Could you check a few things on this model? Use its own coordinates, in mm. A direction names the side the tool comes from. Coordinates: 2 decimals unless noted, no trailing zeros. Order: outer loops, then holes, each group sorted by start corner. A loop starts at its lowest first (then second) coordinate and runs counter-clockwise, first axis right, second up. Notation, with made-up numbers: M 74.5,53 L 119.5,53 A25 ccw 119.5,75 Z; hole C 85.5,30.5 d5. An arc over 180 degrees is marked long. Put each result on its own line as item: value. Start each with the question number.
Autodesk Inventor part; units mm, degrees
ref_plane "YZ Plane" through (0, 0, 0) normal (1, 0, 0) x (0, 1, 0)
ref_plane "XZ Plane" through (0, 0, 0) normal (0, 1, 0) x (-1, 0, 0)
ref_plane "XY Plane" through (0, 0, 0) normal (0, 0, 1) x (1, 0, 0)
sketch "Sketch1" plane through (0, 0, 0) normal (0, 0, 1) x (1, 0, 0)
  line L0 (-33.5, -13) -> (33.5, -13) construction
  line L1 (33.5, -13) -> (33.5, 13) construction
  line L2 (33.5, 13) -> (-33.5, 13) construction
  line L3 (-33.5, 13) -> (-33.5, -13) construction
  line L4 (-33.5, -13) -> (33.5, 13) construction
  line L5 (33.5, -13) -> (-33.5, 13) construction
  arc A0 (-33.5, 19) -> (-39.3825, 11.8182) centre (-33.5, 13) ccw
  arc A1 (-39.3825, -11.8182) -> (-33.5, -19) centre (-33.5, -13) ccw
  arc A2 (33.5, -19) -> (39.3825, -11.8182) centre (33.5, -13) ccw
  arc A3 (39.3825, 11.8182) -> (33.5, 19) centre (33.5, 13) ccw
  arc A4 (-39.3825, -11.8182) -> (-39.3825, 11.8182) centre (-98.207, 0) ccw
  arc A5 (39.3825, 11.8182) -> (39.3825, -11.8182) centre (98.207, 0) ccw
  line L6 (-33.5, 19) -> (33.5, 19)
  line L7 (-33.5, -19) -> (33.5, -19)
  point P0 (0, 0)
  dimension "d0" = 67
  dimension "d1" = 26
  dimension "d2" = 6
  dimension "d3" = 60
extrude "Extrusion1" add sketch "Sketch1" along normal blind 6
sketch "Sketch2" plane through (0, 0, 0) normal (1, 0, 0) x (0, 1, 0)
  line L0 (19, 6) -> (11.8182, 6) construction
  line L1 (19, 6) -> (7, 49)
  line L2 (7, 49) -> (1, 49)
  line L3 (1, 49) -> (-19, 6)
  line L4 (19, 6) -> (11.8182, 6) construction
  line L5 (11.8182, 6) -> (-11.8182, 6) construction
  line L6 (-11.8182, 6) -> (-19, 6) construction
  line L7 (-19, 6) -> (-11.8182, 6) construction
  line L8 (-11.8182, 6) -> (11.8182, 6) construction
  line L9 (11.8182, 6) -> (19, 6) construction
  line L10 (19, 6) -> (-19, 6)
  point P0 (0, 0)
  dimension "d7" = 12
  dimension "d8" = 43
  dimension "d9" = 6
extrude "Extrusion2" add sketch "Sketch2" along normal mid plane 55
sketch "Sketch3" plane through (-27.5, 1, 49) normal (0, 0, 1) x (1, 0, 0)
  line L0 (0, 0) -> (55, 0)
  line L1 (55, 6) -> (55, 0)
  line L2 (0, 6) -> (55, 6)
  line L3 (0, 0) -> (0, 6)
  line L4 (0, 6) -> (55, 6)
  line L5 (61, 18) -> (-6, 18)
  line L6 (4, 6) -> (51, 6)
  line L7 (51, 6) -> (51, 18)
  line L8 (51, 18) -> (4, 18)
  line L9 (4, 18) -> (4, 6)
  line L10 (0, 0) -> (55, 0)
  line L11 (-6, -20) -> (61, -20)
  line L12 (4, 0) -> (51, 0)
  line L13 (51, 0) -> (51, -20)
  line L14 (51, -20) -> (4, -20)
  line L15 (4, -20) -> (4, 0)
  point P0 (27.5, -1)
  dimension "d12" = 4
  dimension "d13" = 4
extrude "Extrusion3" cut sketch "Sketch3" against normal up to surface (43 mm away) contours L0 L13 L11 L15 | L9 L5 L7 L2
sketch "Sketch4" plane through (-23.5, 7, 49) normal (0, 1, 0) x (1, 0, 0)
  arc A0 (36.54, 17.5059) -> (10.46, 17.5059) centre (23.5, 21) ccw
  line L0 (47, 43) -> (0, 43)
  line L1 (57, 49) -> (-10, 49)
  line L2 (36.54, 17.5059) -> (31.8493, 0)
  line L3 (31.8493, 0) -> (15.1507, 0)
  line L4 (15.1507, 0) -> (10.46, 17.5059)
  line L5 (0, 0) -> (47, 0)
  arc A1 (10.46, 17.5059) -> (36.54, 17.5059) centre (23.5, 21) ccw construction
  point P0 (23.5, 49)
  point P1 (23.5, 49)
  point P2 (23.5, 0)
  point P3 (23.5, 49)
  dimension "d16" = 27
  dimension "d17" = 22
  dimension "d18" = 30
extrude "Extrusion4" cut sketch "Sketch4" against normal blind 55
fillet "Fillet1" radius 5 2 edges at (8.3493, 4, 49) (-8.3493, 4, 49)
sketch "Sketch5" plane through (-23.5, 7, 6) normal (0, 1, 0) x (1, 0, 0)
  arc A0 (36.54, -25.4941) -> (10.46, -25.4941) centre (23.5, -22) ccw
  line L0 (8, -6.5) -> (39, -6.5)
  line L1 (39, -6.5) -> (39, -37.5)
  line L2 (39, -37.5) -> (8, -37.5)
  line L3 (8, -37.5) -> (8, -6.5)
  line L4 (8, -6.5) -> (39, -37.5) construction
  line L5 (39, -6.5) -> (8, -37.5) construction
  point P0 (23.5, 6)
  dimension "d22" = 31
  dimension "d23" = 31
hole "Hole1" at (-15.5, 7, 12.5) at (15.5, 7, 12.5) at (15.5, 7, 43.5) at (-15.5, 7, 43.5) direction (0, -1, 0) diameter 4 end through all
sketch "Sketch6" plane through (0, 0, 0) normal (0, 0, -1) x (-1, 0, 0)
  arc A0 (-33.5, -19) -> (-32.6299, -18.9366) centre (-33.5, -13) ccw
  arc A1 (32.6299, -18.9366) -> (-32.6299, -18.9366) centre (0, -241.558) ccw
  arc A2 (32.6299, -18.9366) -> (33.5, -19) centre (33.5, -13) ccw
  line L0 (-33.5, -19) -> (33.5, -19)
  arc A3 (33.5, -19) -> (39.3825, -11.8182) centre (33.5, -13) ccw
  arc A4 (-39.3825, -11.8182) -> (-33.5, -19) centre (-33.5, -13) ccw
  point P0 (0, 0)
  dimension "d31" = 225
extrude "Extrusion5" cut sketch "Sketch6" against normal blind 55
sketch "Sketch7" plane through (0, 0, 0) normal (0, 0, -1) x (-1, 0, 0)
  line L0 (-33.5, -13) -> (33.5, -13) construction
  line L1 (33.5, -13) -> (33.5, 13) construction
  line L2 (33.5, 13) -> (-33.5, 13) construction
  line L3 (-33.5, 13) -> (-33.5, -13) construction
  line L4 (-33.5, -13) -> (33.5, 13) construction
  line L5 (33.5, -13) -> (-33.5, 13) construction
  arc A0 (-39.3825, -11.8182) -> (-32.6299, -18.9366) centre (-33.5, -13) ccw construction
  arc A1 (32.6299, -18.9366) -> (-32.6299, -18.9366) centre (0, -241.558) ccw construction
  arc A2 (32.6299, -18.9366) -> (39.3825, -11.8182) centre (33.5, -13) ccw construction
  arc A3 (39.3825, 11.8182) -> (39.3825, -11.8182) centre (98.207, 0) ccw construction
  arc A4 (39.3825, 11.8182) -> (33.5, 19) centre (33.5, 13) ccw construction
  line L6 (-33.5, 19) -> (33.5, 19) construction
  arc A5 (-33.5, 19) -> (-39.3825, 11.8182) centre (-33.5, 13) ccw construction
  arc A6 (-39.3825, -11.8182) -> (-39.3825, 11.8182) centre (-98.207, 0) ccw construction
  point P0 (0, 0)
  point P1 (0, 0)
  dimension "d34" = 67
  dimension "d35" = 26
hole "Hole2" at (33.5, 13, 0) at (33.5, -13, 0) at (-33.5, -13, 0) at (-33.5, 13, 0) direction (0, 0, 1) diameter 4 depth 14.2 tip angle 118
sketch "Sketch8" plane through (0, 0, 6) normal (0, 0, 1) x (1, 0, 0)
  circle A0 centre (-33.5, -13) radius 2
  circle A1 centre (-33.5, 13) radius 2
  arc A2 (-39.3825, -11.8182) -> (-32.6299, -18.9366) centre (-33.5, -13) ccw
  arc A3 (-27.5, -18.2449) -> (-32.6299, -18.9366) centre (0, -241.558) ccw
  line L0 (-27.5, -18.2449) -> (-27.5, 19)
  line L1 (-27.5, 19) -> (-33.5, 19)
  arc A4 (-33.5, 19) -> (-39.3825, 11.8182) centre (-33.5, 13) ccw
  arc A5 (-39.3825, -11.8182) -> (-39.3825, 11.8182) centre (-98.207, 0) ccw
  circle A6 centre (33.5, 13) radius 2
  circle A7 centre (33.5, -13) radius 2
  arc A8 (32.6299, -18.9366) -> (39.3825, -11.8182) centre (33.5, -13) ccw
  arc A9 (39.3825, 11.8182) -> (39.3825, -11.8182) centre (98.207, 0) ccw
  arc A10 (39.3825, 11.8182) -> (33.5, 19) centre (33.5, 13) ccw
  line L2 (33.5, 19) -> (27.5, 19)
  line L3 (27.5, 19) -> (27.5, -18.2449)
  arc A11 (32.6299, -18.9366) -> (27.5, -18.2449) centre (0, -241.558) ccw
  line L4 (-30.1519, 11.067) -> (-33.5, 9.134)
  line L5 (-33.5, 9.134) -> (-36.8481, 11.067)
  line L6 (-36.8481, 11.067) -> (-36.8481, 14.933)
  line L7 (-36.8481, 14.933) -> (-33.5, 16.866)
  line L8 (-33.5, 16.866) -> (-30.1519, 14.933)
  line L9 (-30.1519, 14.933) -> (-30.1519, 11.067)
  line L10 (-30.1519, -14.933) -> (-33.5, -16.866)
  line L11 (-33.5, -16.866) -> (-36.8481, -14.933)
  line L12 (-36.8481, -14.933) -> (-36.8481, -11.067)
  line L13 (-36.8481, -11.067) -> (-33.5, -9.134)
  line L14 (-33.5, -9.134) -> (-30.1519, -11.067)
  line L15 (-30.1519, -11.067) -> (-30.1519, -14.933)
  line L16 (36.8481, -14.933) -> (33.5, -16.866)
  line L17 (33.5, -16.866) -> (30.1519, -14.933)
  line L18 (30.1519, -14.933) -> (30.1519, -11.067)
  line L19 (30.1519, -11.067) -> (33.5, -9.134)
  line L20 (33.5, -9.134) -> (36.8481, -11.067)
  line L21 (36.8481, -11.067) -> (36.8481, -14.933)
  line L22 (36.8481, 11.067) -> (33.5, 9.134) construction
  line L23 (33.5, 9.134) -> (30.1519, 11.067) construction
  line L24 (30.1519, 11.067) -> (30.1519, 14.933) construction
  line L25 (30.1519, 14.933) -> (33.5, 16.866) construction
  line L26 (33.5, 16.866) -> (36.8481, 14.933) construction
  line L27 (36.8481, 14.933) -> (36.8481, 11.067) construction
  arc A12 (30.1519, 14.933) -> (33.5, 16.866) centre (30.075, 18.9323) ccw
  arc A13 (33.5, 16.866) -> (36.8481, 14.933) centre (36.925, 18.9323) ccw
  arc A14 (36.8481, 11.067) -> (33.5, 9.134) centre (36.925, 7.0677) ccw
  arc A15 (33.5, 9.134) -> (30.1519, 11.067) centre (30.075, 7.0677) ccw
  arc A16 (30.1519, 11.067) -> (30.1519, 14.933) centre (26.65, 13) ccw
  arc A17 (36.8481, 14.933) -> (36.8481, 11.067) centre (40.35, 13) ccw
  point P0 (0, 0)
  dimension "d44" = 6.6962
  dimension "d47" = 4
  dimension "d48" = 4
  dimension "d49" = 4
  dimension "d50" = 4
  dimension "d51" = 4
  dimension "d52" = 4
  dimension "d53" = 5.7
extrude "Extrusion6" cut sketch "Sketch8" against normal blind 3 contours A12 A13 A17 A14 A15 A16
pattern_linear "Rectangular Pattern1" count 2 spacing 67 along (-1, 0, 0) count 2 spacing 26 along (0, -1, 0) of "Extrusion6"
equation "\"d13\" = d12"
properties part number "Y Motor Mount" material "ABS Plastic"
Item 1: For pin 1 Ø7.5 at (x, y) = (34.5, 14) entering from +Z; pin 2 Ø13 at (y, z) = (12, 34) entering from +X; pin 3 Ø9.5 at (y, z) = (14.5, 36.5) entering from -X, each with a flat end and sliding along its axis, tell me the tip position at first contact or that it passes through.
Item 2: I need wall thicknesses on probe 1 along X at (y, z) = (13, 1.05); probe 2 along Y at (x, z) = (33.5, 1.25); probe 3 along Z at (x, y) = (-15.5, 5.1). Which ranges of each line are inside material? Lowest first, please.
Item 3: If we section it at B-B on x = 0: Write out the boundary of the cut face in (y, z), then the cut area to 3 significant figures.
Item 4: If we section it at A-A on y = 13: Write out the boundary of the cut face in (x, z), then the cut area to 3 significant figures.
Item 5: For faces 4 (the flat face through (32.7, 15, 3)), 5 (the flat face through (0, 13, 6)), 6 (the cylindrical face through (35.452, 12.566, 1.521)), which set-ups out of +Z, -Z, +X, -X, +Y, -Y let a thin tool reach every point of the face, with its end or its side?
Item 6: If we mould it in two halves opening along Z, with no side actions, what happens to faces 1 (the cylindrical face through (13.517, 3.958, 43.24)), 2 (the cylindrical face through (-31.548, -13.434, 1.521)), 3 (the flat face through (-34.3, -11, 3))? For each: released by +Z, released by -Z, zero draft, split by the parting line, or undercut.
Item 7: If we section it at D-D on z = 28: Write out the boundary of the cut face in (x, y), then the cut area to 3 significant figures.
Item 8: If we section it at C-C on z = 12.5: Write out the boundary of the cut face in (x, y).
Geometry check:
1. pin 1: stops at z = 6
1. pin 2: stops at x = 27.5
1. pin 3: stops at x = -27.5
2. probe 1: x = -39.5 to -35.5, -31.5 to 31.5, 35.5 to 39.5
2. probe 2: y = -19 to -15, -11 to 11, 15 to 19
2. probe 3: z = 0 to 10.5, 14.5 to 41.5, 45.5 to 49
3. outline: M -16.56,0 L 19,0 L 19,6 L 7,6 L 7,14.5 L 1,14.5 L 1,6 L -16.56,6 Z
3. area: 264 mm²
4. outline: M -39.5,0 L -35.5,0 L -35.5,3 L -36.35,3 L -36.35,6 L -39.5,6 Z; M -31.5,0 L 31.5,0 L 31.5,3 L 30.65,3 L 30.65,6 L 27.5,6 L 27.5,27.5 L 23.5,27.5 L 23.5,6 L -23.5,6 L -23.5,27.5 L -27.5,27.5 L -27.5,6 L -30.65,6 L -30.65,3 L -31.5,3 Z; M 35.5,0 L 39.5,0 L 39.5,6 L 36.35,6 L 36.35,3 L 35.5,3 Z
4. area: 588 mm²
5. face 4: +Z
5. face 5: +Z, +Y
5. face 6: +Z, -Z
6. face 1: undercut
6. face 2: zero draft
6. face 3: released by +Z
7. outline: M -27.5,-8.77 L -23.5,-8.77 L -23.5,1 L -13.5,1 L -13.5,7 L -23.5,7 L -23.5,12.86 L -27.5,12.86 Z; M 13.5,1 L 23.5,1 L 23.5,-8.77 L 27.5,-8.77 L 27.5,12.86 L 23.5,12.86 L 23.5,7 L 13.5,7 Z
7. area: 293 mm²
8. outline: M -27.5,-15.98 L -23.5,-15.98 L -23.5,1 L -17.5,1 L -17.5,7 L -23.5,7 L -23.5,17.19 L -27.5,17.19 Z; M -13.5,1 L 13.5,1 L 13.5,7 L -13.5,7 Z; M 17.5,1 L 23.5,1 L 23.5,-15.98 L 27.5,-15.98 L 27.5,17.19 L 23.5,17.19 L 23.5,7 L 17.5,7 Z
